The model under review builds one solid part; all positions refer to its coordinate system, in mm. Coordinates: 2 decimals unless noted, no trailing zeros. Loops run counter-clockwise (first coordinate to the right, second up) from the corner with the lowest first, then second, coordinate; pieces in that order, holes last. Notation, with made-up numbers: M -8.75,75.5 L 16.25,75.5 A8 cw 16.25,88.5 Z; hole C -5,62.5 d4. An arc over 180 degrees is marked long. Use CSV: the item, a comma, the result in double quotes. Start each with the question number.
1. Add section A-A, the plane z = 0. Write out the cut boundary in (x, y).
2. Clearance check with flat-ended pins moving along their axes: P1, Ø4, axis at y = 3.5, z = 4, coming from the +X side; P2, Ø0.8, axis at x = -26, y = 0, coming from the +Z side; P3, Ø1.6, axis at y = -0.5, z = -0.5, coming from the +X side. State where each tip first meets the part, or that it passes through.
3. Add section B-B, the plane x = 79.5. Write out the cut boundary in (y, z), then the cut area to 3 significant figures.
4. For L1, parallel to Y at x = 35.5, z = 3.75; L2, parallel to X at y = 3.5, z = 4.5, list the stretches that pass through material, from the lowest coordinate up.
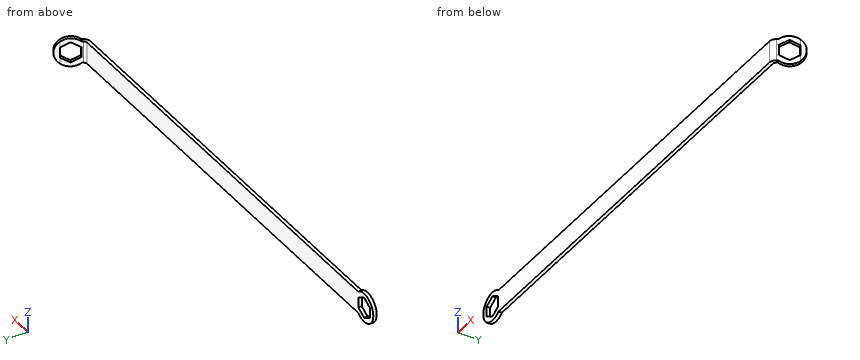
from build123d import *

# Parameters (mm, degrees)
SKETCH1_W              = 190.5125
SKETCH1_H              = 9.6
BOSS_EXTRUDE1_DEPTH    = 0.75
SKETCHED_START         = 85.719592776
SKETCHED_BEND1_DEPTH   = 7.280407224
SKETCHED_START_2       = -7
SKETCHED_BEND1_2_DEPTH = 14
SKETCHED_START_3       = -6.35
SKETCHED_BEND1_3_DEPTH = 4.058641119
SKETCHED_START_4       = 2.291358881
SKETCHED_BEND1_4_DEPTH = 4.058641119
SKETCHED_START_5       = -3.11420605
SKETCHED_BEND1_5_DEPTH = 6.2284121
SKETCHED_START_6       = 81.780241505
SKETCHED_BEND1_6_DEPTH = 10.219758495
SKETCHED_START_7       = 79
SKETCHED_BEND1_7_DEPTH = 2.780241505
SKETCHED_START_8       = 80.280241505
SKETCHED_BEND1_8_DEPTH = 1.5


with BuildPart() as part:
    # Sketch1 → Boss-Extrude1 (new, symmetric)
    # profile 1 of 3: a face of its own
    with BuildSketch(Plane(origin=(0, 0, 0), x_dir=(1, 0, 0), z_dir=(0, 1, 0))):
        with BuildLine():
            Line((-95.25625, 4.8), (-95.25625, -4.8))
            ThreePointArc((-95.25625, -4.8), (-105.763472631, 0), (-95.25625, 4.8))
        make_face()
        Polygon((-103.382222631, -2.291358881), (-99.413472631, -4.582717762), (-95.444722631, -2.291358881), (-95.444722631, 2.291358881), (-99.413472631, 4.582717762), (-103.382222631, 2.291358881), align=None, mode=Mode.SUBTRACT)
    # profile 2 of 3: a face of its own
    with BuildSketch(Plane(origin=(0, 0, 0), x_dir=(1, 0, 0), z_dir=(0, 1, 0))):
        Rectangle(SKETCH1_W, SKETCH1_H)
    # profile 3 of 3: a face of its own
    with BuildSketch(Plane(origin=(0, 0, 0), x_dir=(1, 0, 0), z_dir=(0, 1, 0))):
        with BuildLine():
            Line((95.25625, 4.8), (95.25625, -4.8))
            ThreePointArc((95.25625, -4.8), (105.763472631, 0), (95.25625, 4.8))
        make_face()
        Polygon((95.444722631, -2.291358881), (99.413472631, -4.582717762), (103.382222631, -2.291358881), (103.382222631, 2.291358881), (99.413472631, 4.582717762), (95.444722631, 2.291358881), align=None, mode=Mode.SUBTRACT)
    extrude(amount=BOSS_EXTRUDE1_DEPTH, both=True)

    # Sketched Bend1: read off the stored shape, not the designer's step
    # Sketched Bend1 outline → Sketched Bend1 (cut)
    with BuildSketch(Plane(origin=(0, 0, 0), x_dir=(0.49999999999999767, 0.86602540378444, 0), z_dir=(0.8660254037844399, -0.49999999999999795, 0)).offset(SKETCHED_START)):
        Polygon((48.903772606, 2.291358881), (48.903772606, -2.291358881), (52.872522606, -4.582717762), (56.841272606, -2.291358881), (56.841272606, 2.291358881), (52.872522606, 4.582717762), align=None)
    extrude(amount=SKETCHED_BEND1_DEPTH, mode=Mode.SUBTRACT)

    # Sketched Bend1 2 outline → Sketched Bend1 2 (cut)
    with BuildSketch(Plane.XY.offset(SKETCHED_START_2)):
        with BuildLine():
            Line((95.444722631, 0.75), (94.864701597, 0.75))
            ThreePointArc((94.864701597, 0.75), (93.766625385, -0.348076211), (92.266625385, -0.75))
            Line((92.266625385, -0.75), (95.444722631, -0.75))
            Line((95.444722631, -0.75), (95.444722631, 0.75))
        make_face()
    extrude(amount=SKETCHED_BEND1_2_DEPTH, mode=Mode.SUBTRACT)

    # Sketched Bend1 3 outline → Sketched Bend1 3 (add)
    with BuildSketch(Plane.XY.offset(SKETCHED_START_3)):
        with BuildLine():
            Line((99.244402974, 8.335865308), (97.945364869, 9.085865308))
            Line((97.945364869, 9.085865308), (93.565663491, 1.5))
            ThreePointArc((93.565663491, 1.5), (93.016625385, 0.950961894), (92.266625385, 0.75))
            Line((92.266625385, 0.75), (94.864701597, 0.75))
            Line((94.864701597, 0.75), (99.244402974, 8.335865308))
        make_face()
    extrude(amount=SKETCHED_BEND1_3_DEPTH)

    # Sketched Bend1 4 outline → Sketched Bend1 4 (add)
    with BuildSketch(Plane.XY.offset(SKETCHED_START_4)):
        with BuildLine():
            Line((99.244402974, 8.335865308), (97.945364869, 9.085865308))
            Line((97.945364869, 9.085865308), (93.565663491, 1.5))
            ThreePointArc((93.565663491, 1.5), (93.016625385, 0.950961894), (92.266625385, 0.75))
            Line((92.266625385, 0.75), (94.864701597, 0.75))
            Line((94.864701597, 0.75), (99.244402974, 8.335865308))
        make_face()
    extrude(amount=SKETCHED_BEND1_4_DEPTH)

    # Sketched Bend1 5 outline → Sketched Bend1 5 (add)
    with BuildSketch(Plane.XY.offset(SKETCHED_START_5)):
        with BuildLine():
            Line((94.864701597, 0.75), (95.275652974, 1.461788665))
            Line((95.275652974, 1.461788665), (93.976614869, 2.211788665))
            Line((93.976614869, 2.211788665), (93.565663491, 1.5))
            ThreePointArc((93.565663491, 1.5), (93.016625385, 0.950961894), (92.266625385, 0.75))
            Line((92.266625385, 0.75), (94.864701597, 0.75))
        make_face()
    extrude(amount=SKETCHED_BEND1_5_DEPTH)

    # Sketched Bend1 6 outline → Sketched Bend1 6 (cut)
    with BuildSketch(Plane(origin=(0, 0, 0), x_dir=(0.49999999999999767, 0.86602540378444, 0), z_dir=(0.8660254037844399, -0.49999999999999795, 0)).offset(SKETCHED_START_6)):
        with BuildLine():
            Line((48.903772606, -2.29135888), (45, -0.037514714))
            Line((45, -0.037514714), (45, -6.35))
            Line((45, -6.35), (52.872522564, -6.35))
            ThreePointArc((52.872522564, -6.35), (54.047030124, -6.240435248), (55.181007092, -5.915521902))
            Line((55.181007092, -5.915521902), (52.872522606, -4.582717762))
            Line((52.872522606, -4.582717762), (48.903772606, -2.29135888))
        make_face()
        with BuildLine():
            Line((45, 0.037514714), (48.903772606, 2.29135888))
            Line((48.903772606, 2.29135888), (52.872522606, 4.582717762))
            Line((52.872522606, 4.582717762), (55.181007092, 5.915521902))
            ThreePointArc((55.181007092, 5.915521902), (54.047030182, 6.240435237), (52.872522681, 6.35))
            Line((52.872522681, 6.35), (45, 6.35))
            Line((45, 6.35), (45, 0.037514714))
        make_face()
    extrude(amount=SKETCHED_BEND1_6_DEPTH, mode=Mode.SUBTRACT)

    # Sketched Bend1 7 outline → Sketched Bend1 7 (cut)
    with BuildSketch(Plane(origin=(0, 0, 0), x_dir=(0.49999999999999767, 0.86602540378444, 0), z_dir=(0.8660254037844399, -0.49999999999999795, 0)).offset(SKETCHED_START_7)):
        Polygon((56.841272607, -2.291358881), (48.903772606, -2.291358881), (52.872522606, -4.582717762), align=None)
        Polygon((48.903772606, 2.291358881), (56.841272607, 2.291358881), (52.872522606, 4.582717762), align=None)
        with BuildLine():
            Line((56.841272606, -6.35), (56.841272606, -4.956967161))
            ThreePointArc((56.841272606, -4.956967161), (54.975586842, -5.991629229), (52.872522564, -6.35))
            Line((52.872522564, -6.35), (56.841272606, -6.35))
        make_face()
        with BuildLine():
            Line((48.715299976, -4.8), (45, -4.8))
            Line((45, -4.8), (45, -6.35))
            Line((45, -6.35), (52.872522564, -6.35))
            ThreePointArc((52.872522564, -6.35), (50.654133531, -5.949894949), (48.715299976, -4.8))
        make_face()
        with BuildLine():
            Line((56.841272606, 4.956967161), (56.841272606, 6.35))
            Line((56.841272606, 6.35), (52.872522681, 6.35))
            ThreePointArc((52.872522681, 6.35), (54.975586897, 5.99162921), (56.841272606, 4.956967161))
        make_face()
        with BuildLine():
            Line((45, 6.35), (45, 4.8))
            Line((45, 4.8), (48.715299976, 4.8))
            ThreePointArc((48.715299976, 4.8), (50.654133586, 5.94989497), (52.872522681, 6.35))
            Line((52.872522681, 6.35), (45, 6.35))
        make_face()
    extrude(amount=SKETCHED_BEND1_7_DEPTH, mode=Mode.SUBTRACT)

    # Sketched Bend1 8 outline → Sketched Bend1 8 (add)
    with BuildSketch(Plane(origin=(0, 0, 0), x_dir=(0.49999999999999767, 0.86602540378444, 0), z_dir=(0.8660254037844399, -0.49999999999999795, 0)).offset(SKETCHED_START_8)):
        with BuildLine():
            Line((56.841272606, 4.956967161), (56.841272606, -4.956967161))
            ThreePointArc((56.841272606, -4.956967161), (59.222522606, 0), (56.841272606, 4.956967161))
        make_face()
    extrude(amount=SKETCHED_BEND1_8_DEPTH)


solid = part.part
Computed:
1,outline,"M -105.76,-0.75 L -103.38,-0.75 L -103.38,0.75 L -105.76,0.75 Z; M -95.44,-0.75 L 92.27,-0.75 A3 ccw 94.86,0.75 L 95.28,1.46 L 93.98,2.21 L 93.57,1.5 A1.5 cw 92.27,0.75 L -95.44,0.75 Z; M 97.95,9.09 L 99.24,8.34 L 100.44,10.4 L 99.14,11.15 Z"
2,P1,"stops at x = 97.6"
2,P2,"stops at z = 4.8"
2,P3,"stops at x = 94.55"
3,outline,"M -0.75,-4.8 L 0.75,-4.8 L 0.75,4.8 L -0.75,4.8 Z"
3,area,"14.4 mm^2"
4,L1,"y = -0.75 to 0.75"
4,L2,"x = 94.72 to 96.45"
